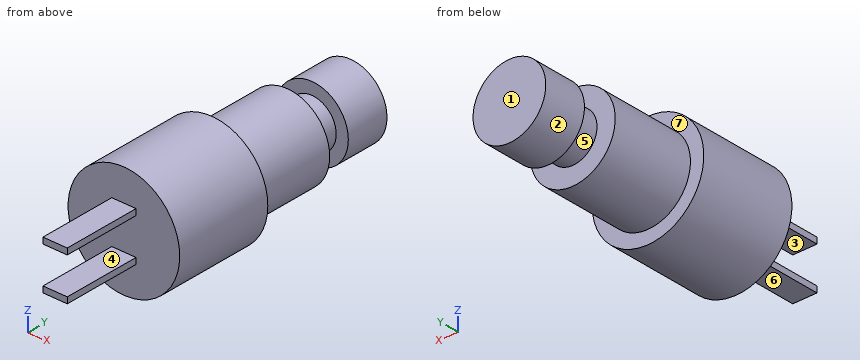
from build123d import *

# Parameters (mm, degrees)
SKETCH_2_W        = 2
SKETCH_2_H        = 0.5
EXTRUDE_795_DEPTH = 6.4


with BuildPart() as part:
    # Эскиз1 → Revolve 542 (revolve)
    with BuildSketch(Plane.XY):
        Polygon((0, 0), (0, 21.1), (3, 21.1), (3, 17.5), (2, 17.5), (2, 15.2), (3.5, 15.2), (3.5, 8.2), (4.6, 8.2), (4.6, 0), align=None)
    revolve(axis=Axis((0, 0, 0), (0, 1, 0)))

    # Эскиз2 → Extrude 795 (add)
    with BuildSketch(Plane.XZ):
        with Locations((0, 1.75)):
            Rectangle(SKETCH_2_W, SKETCH_2_H)
        with Locations((0, -1.75)):
            Rectangle(SKETCH_2_W, SKETCH_2_H)
    extrude(amount=EXTRUDE_795_DEPTH)


solid = part.part
Work out the finished part from the listing and answer in its coordinate system (mm). Face numbers are marked on the shaded views. A direction names the side the tool comes from. Round coordinates to 2 decimals unless told otherwise and drop trailing zeros. Loops run counter-clockwise (first coordinate to the right, second up) from the corner with the lowest first, then second, coordinate; pieces in that order, holes last. Notation, with made-up numbers: (-34, 48) - (-24, 48) arc R23 ccw to (-24, 73) - close; hole circle Ø8 at (-25.5, 56). An arc over 180 degrees is marked (long way). Use one line per item in the form item = value. Start each with the question number.
(1) Which of the six approach directions +Z, -Z, +X, -X, +Y, -Y give full straight-line access (tool end or side, diameter ignored) to the marked faces 5, 6 and 7?
(2) Determine the mould class of the marked faces 1, 2, 3 and 4 for opening direction Z: +Z half, -Z half, draft (parallel to the pull), parting line (faces both ways), or undercut.
(3) Consider line 1 (Y direction, x = -3.75, z = 0.5); line 2 (Y direction, x = 1, z = -0.75); line 3 (Z direction, x = -0.75, y = 11.5). Determine where each line is inside the solid, lowest interval first.
(4) Find section D-D on z = 0. Determine the outline of the cut face in (x, y), and give its area (3 significant figures).
(5) Flat-ended cylindrical pins translate along their axes: P1, Ø5, axis at x = -3.5, y = 14, coming from the +Z side; P2, Ø4, axis at y = 11.5, z = -3, coming from the +X side; P3, Ø1.5, axis at x = -3, z = -1.5, coming from the -Y side. Find the tip coordinate at first contact, or state that the pin passes through.
(6) Find section B-B on z = -2.5. Determine the outline of the cut face in (x, y).
(7) Find section C-C on x = 0. Determine the outline of the cut face in (y, z).
(8) Find section A-A on y = -2.5. Determine the outline of the cut face in (x, z), and give its area (3 significant figures).
Answer list:
q1.face_5 = none
q1.face_6 = -Z, +X, -X, -Y
q1.face_7 = +Y
q2.face_1 = draft
q2.face_2 = parting line
q2.face_3 = undercut
q2.face_4 = undercut
q3.line_1 = 0 to 8.2
q3.line_2 = 0 to 21.1
q3.line_3 = -3.42 to 3.42
q4.outline = (-4.6, 0) - (4.6, 0) - (4.6, 8.2) - (3.5, 8.2) - (3.5, 15.2) - (2, 15.2) - (2, 17.5) - (3, 17.5) - (3, 21.1) - (-3, 21.1) - (-3, 17.5) - (-2, 17.5) - (-2, 15.2) - (-3.5, 15.2) - (-3.5, 8.2) - (-4.6, 8.2) - close
q4.area = 155 mm^2
q5.P1 = 3.35
q5.P2 = 3.35
q5.P3 = 0
q6.outline = (-3.86, 0) - (3.86, 0) - (3.86, 8.2) - (2.45, 8.2) - (2.45, 15.2) - (-2.45, 15.2) - (-2.45, 8.2) - (-3.86, 8.2) - close; (-1.66, 17.5) - (1.66, 17.5) - (1.66, 21.1) - (-1.66, 21.1) - close
q7.outline = (-6.4, -2) - (0, -2) - (0, -4.6) - (8.2, -4.6) - (8.2, -3.5) - (15.2, -3.5) - (15.2, -2) - (17.5, -2) - (17.5, -3) - (21.1, -3) - (21.1, 3) - (17.5, 3) - (17.5, 2) - (15.2, 2) - (15.2, 3.5) - (8.2, 3.5) - (8.2, 4.6) - (0, 4.6) - (0, 2) - (-6.4, 2) - (-6.4, 1.5) - (0, 1.5) - (0, -1.5) - (-6.4, -1.5) - close
q8.outline = (-1, -2) - (1, -2) - (1, -1.5) - (-1, -1.5) - close; (-1, 1.5) - (1, 1.5) - (1, 2) - (-1, 2) - close
q8.area = 2.00 mm^2
